Geometry check sheet. Reference: the model listing, model coordinates, mm. A direction names the side the tool comes from. Give positions to 0.01 mm unless a question says otherwise; leave off trailing zeros. Loops run counter-clockwise (first coordinate to the right, second up) from the corner with the lowest first, then second, coordinate; pieces in that order, holes last. Notation, with made-up numbers: (-22, -35.5) - (0, -35.5) arc R27 ccw to (0, -8.5) - close; hole circle Ø3 at (-24, 60.5). An arc over 180 degrees is marked (long way). Use a Markdown table: item, result. Add a question column.
1. Cross-section at A-A on z = 1. Enter the section's corners in (x, y).
2. Cross-section at D-D on x = 15. Enter the section's corners in (y, z).
3. Draft check along X on faces 1 (the flat face through (9, 18, 4)), 2 (the cylindrical face through (19.125, 1.036, 6.028)), 3 (the flat face through (14, 20, 4)), 4 (the flat face through (28.9, 10, 5)). Enter one of: pulls with the +X half, pulls with the -X half, needs draft (parallel to the pull), parting line crosses it, or undercut.
4. Material ranges on L1, parallel to Y at x = 19.45, z = 6.65; L2, parallel to Y at x = 14.25, z = 1.75; L3, parallel to Y at x = 10.25, z = 5.5, recorded low to high.
5. Set-up check for faces 5 (the flat face through (26, 10, 7.9)), 6 (the flat face through (14, 17, 0)), 7 (the flat face through (2, 10, 7.9)), 8 (the cylindrical face through (9.125, 1.036, 6.028)), 9 (the flat face through (14, 10, 4.5)): record each of +Z, -Z, +X, -X, +Y, -Y from which the full face is reachable in a straight line by a thin tool's end or side.
6. Cross-section at B-B on x = 19.45. Enter the section's corners in (y, z).
7. Cross-section at C-C on y = 17.5. Enter the section's corners in (x, z), and give its area (3 significant figures).
8. Depth check by flat-ended pin: P1, Ø0.9, axis at x = 20, y = 17.5, coming from the +Z side; P2, Ø4.5, axis at x = 15.5, y = 9, coming from the -Z side; P3, Ø2.5, axis at x = 3.5, y = 9, coming from the +Z side. Enter the tip coordinate at first touch or a pass-through.
from build123d import *

# Parameters (mm, degrees)
SKETCH002_W     = 28.9
SKETCH002_H     = 20
PAD001_DEPTH    = 8
SKETCH003_W     = 9
SKETCH003_H     = 4.5
POCKET001_DEPTH = 28.9
SKETCH004_R     = 1.5
POCKET002_DEPTH = 4
SKETCH005_W     = 5
SKETCH005_H     = 20
POCKET003_DEPTH = 0.1


with BuildPart() as part:
    # Sketch002 → Pad001 (new body)
    with BuildSketch(Plane.XY):
        with Locations((14.45, 10)):
            Rectangle(SKETCH002_W, SKETCH002_H)
    extrude(amount=PAD001_DEPTH)

    # Sketch003 (on Face4 of Pad001) → Pocket001 (cut)
    with BuildSketch(Plane(origin=(0, 0, 0), x_dir=(0, -1, 0), z_dir=(-1, 0, 0))):
        with Locations((-10, 2.25)):
            Rectangle(SKETCH003_W, SKETCH003_H)
    extrude(amount=-POCKET001_DEPTH, mode=Mode.SUBTRACT)

    # Sketch004 (on Face5 of Pocket001) → Pocket002 (cut)
    with BuildSketch(Plane.XY.offset(8)):
        with Locations((9.45, 17.5)):
            Circle(SKETCH004_R)
        with Locations((19.45, 17.5)):
            Circle(SKETCH004_R)
        with Locations((19.45, 2.5)):
            Circle(SKETCH004_R)
        with Locations((9.45, 2.5)):
            Circle(SKETCH004_R)
    extrude(amount=-POCKET002_DEPTH, mode=Mode.SUBTRACT)

    # Sketch005 (on Face5 of Pocket002) → Pocket003 (cut)
    with BuildSketch(Plane.XY.offset(8)):
        with Locations((2.5, 10)):
            Rectangle(SKETCH005_W, SKETCH005_H)
        with Locations((26.4, 10)):
            Rectangle(SKETCH005_W, SKETCH005_H)
    extrude(amount=-POCKET003_DEPTH, mode=Mode.SUBTRACT)


solid = part.part
Values found:
| question | item | result |
|---|---|---|
| 1 | outline | (0, 0) - (28.9, 0) - (28.9, 5.5) - (0, 5.5) - close; (0, 14.5) - (28.9, 14.5) - (28.9, 20) - (0, 20) - close |
| 2 | outline | (0, 0) - (5.5, 0) - (5.5, 4.5) - (14.5, 4.5) - (14.5, 0) - (20, 0) - (20, 8) - (0, 8) - close |
| 3 | face 1 | undercut |
| 3 | face 2 | undercut |
| 3 | face 3 | needs draft |
| 3 | face 4 | pulls with the +X half |
| 4 | L1 | y = 0 to 1, 4 to 16, 19 to 20 |
| 4 | L2 | y = 0 to 5.5, 14.5 to 20 |
| 4 | L3 | y = 0 to 1.23, 3.77 to 16.23, 18.77 to 20 |
| 5 | face 5 | +Z, +X, +Y, -Y |
| 5 | face 6 | -Z, +X, -X, +Y, -Y |
| 5 | face 7 | +Z, -X, +Y, -Y |
| 5 | face 8 | +Z |
| 5 | face 9 | -Z, +X, -X |
| 6 | outline | (0, 0) - (5.5, 0) - (5.5, 4.5) - (14.5, 4.5) - (14.5, 0) - (20, 0) - (20, 8) - (19, 8) - (19, 4) - (16, 4) - (16, 8) - (4, 8) - (4, 4) - (1, 4) - (1, 8) - (0, 8) - close |
| 7 | outline | (0, 0) - (28.9, 0) - (28.9, 7.9) - (23.9, 7.9) - (23.9, 8) - (20.95, 8) - (20.95, 4) - (17.95, 4) - (17.95, 8) - (10.95, 8) - (10.95, 4) - (7.95, 4) - (7.95, 8) - (5, 8) - (5, 7.9) - (0, 7.9) - close |
| 7 | area | 206 mm2 |
| 8 | P1 | stops at z = 4 |
| 8 | P2 | stops at z = 4.5 |
| 8 | P3 | stops at z = 7.9 |
